from build123d import *

# Parameters (mm, degrees)
SKETCH1_W          = 1330.325
SKETCH1_H          = 882.65
EXTRUDE1_DEPTH     = 4.7625
SKETCH2_R          = 6.35
CUT_EXTRUDE1_DEPTH = 5.7625
SKETCH3_R          = 25.4
CUT_EXTRUDE2_DEPTH = 5.7625


with BuildPart() as part:
    # Sketch1 → Extrude1 (new body)
    with BuildSketch(Plane.XY):
        with Locations((0, 638.175)):
            Rectangle(SKETCH1_W, SKETCH1_H)
    extrude(amount=EXTRUDE1_DEPTH)

    # Sketch2 → Cut-Extrude1 (cut, through all)
    with BuildSketch(Plane.XY.offset(4.7625)):
        with Locations((514.35, 956.31)):
            Circle(SKETCH2_R)
        with Locations((514.35, 562.61)):
            Circle(SKETCH2_R)
        with Locations((514.35, 219.71)):
            Circle(SKETCH2_R)
        with Locations((-514.35, 219.71)):
            Circle(SKETCH2_R)
        with Locations((-514.35, 562.61)):
            Circle(SKETCH2_R)
        with Locations((-514.35, 956.31)):
            Circle(SKETCH2_R)
    extrude(amount=-CUT_EXTRUDE1_DEPTH, mode=Mode.SUBTRACT)

    # Sketch3 → Cut-Extrude2 (cut, through all)
    with BuildSketch(Plane.XY.offset(4.7625)):
        with Locations((304.8, 1003.3)):
            Circle(SKETCH3_R)
        with Locations((-304.8, 1003.3)):
            Circle(SKETCH3_R)
    extrude(amount=-CUT_EXTRUDE2_DEPTH, mode=Mode.SUBTRACT)


solid = part.part
Could you check a few things on this model? Use its own coordinates, in mm. Give positions to 0.01 mm unless a question says otherwise; leave off trailing zeros. Order: outer loops, then holes, each group sorted by start corner. A loop starts at its lowest first (then second) coordinate and runs counter-clockwise, first axis right, second up.
1. Thinking about a two-plate mould opening in Y: for faces 1 (the cylindrical face through (299.294, 978.504, 2.415)), 2 (the flat face through (-9, 644, 4.762)), which applies, +Y half, -Y half, draft (parallel to the pull), parting line (faces both ways), or undercut?
Answers below:
face 1: undercut
face 2: draft
2. I need wall thicknesses on L1, parallel to X at y = 956.31, z = 3.6; L2, parallel to Y at x = -514.35, z = 2.15; L3, parallel to Y at x = 513.5, z = 0.25. Which ranges of each line are inside material? Lowest first, please.
Answers below:
L1: x = -665.16 to -520.7, -508 to 508, 520.7 to 665.16
L2: y = 196.85 to 213.36, 226.06 to 556.26, 568.96 to 949.96, 962.66 to 1079.5
L3: y = 196.85 to 213.42, 226 to 556.32, 568.9 to 950.02, 962.6 to 1079.5
3. Suppose I cut it at B-B (x = 304.8). Write out the boundary of the cut face in (y, z), plus the area to 3 significant figures.
Answers below:
outline: (196.85, 0) - (977.9, 0) - (977.9, 4.76) - (196.85, 4.76) - close; (1028.7, 0) - (1079.5, 0) - (1079.5, 4.76) - (1028.7, 4.76) - close
area: 3,960 mm2
4. Suppose I cut it at A-A (y = 1003.3). Write out the boundary of the cut face in (x, z).
Answers below:
outline: (-665.16, 0) - (-330.2, 0) - (-330.2, 4.76) - (-665.16, 4.76) - close; (-279.4, 0) - (279.4, 0) - (279.4, 4.76) - (-279.4, 4.76) - close; (330.2, 0) - (665.16, 0) - (665.16, 4.76) - (330.2, 4.76) - close
